```python
from build123d import *

# Parameters (mm, degrees)
SKETCH1_R                                         = 40
SKETCH1_R_2                                       = 19
BOSS_EXTRUDE1_DEPTH                               = 5
SKETCH2_R                                         = 40
SKETCH2_R_2                                       = 27
BOSS_EXTRUDE2_DEPTH                               = 4
SKETCH3_R                                         = 40
SKETCH3_R_2                                       = 32
BOSS_EXTRUDE3_DEPTH                               = 3
BOSS_EXTRUDE4_REACH                               = 92.244
BOSS_EXTRUDE4_END_RADIUS                          = 40
SKETCH6_W                                         = 12
SKETCH6_H                                         = 80
BOSS_EXTRUDE4_DIRECTION_2_DEPTH                   = 20
SKETCH9_W                                         = 60
SKETCH9_H                                         = 8
BOSS_EXTRUDE5_DEPTH                               = 82
SKETCH19_R                                        = 2.7
SKETCH19_W                                        = 18
SKETCH19_H                                        = 26
CUT_EXTRUDE8_DEPTH                                = 12
SKETCH5_R                                         = 1.4
SKETCH5_R_2                                       = 1.375
CUT_EXTRUDE1_HOLE_DEPTH                           = 149.013512897
CUT_EXTRUDE9_REALITY_DEPTH                        = 148.74302014
CUT_EXTRUDE9_REALITY_DEPTH_BACK                   = 148.74302014
CBORE_FOR_M5_HEX_HEAD_BOLT1_D                     = 5.4
CBORE_FOR_M5_HEX_HEAD_BOLT1_DEPTH                 = 17
CBORE_FOR_M5_HEX_HEAD_BOLT1_CBORE_D               = 8.4
CBORE_FOR_M5_HEX_HEAD_BOLT1_CBORE_DEPTH           = 5
CSK_FOR_M2_5_FLAT_HEAD_MACHINE_SCREW1_D           = 2.8
CSK_FOR_M2_5_FLAT_HEAD_MACHINE_SCREW1_CSINK_D     = 5.1
CSK_FOR_M2_5_FLAT_HEAD_MACHINE_SCREW1_CSINK_ANGLE = 90
FILLET1_5MM_R                                     = 5
FILLET2_2MM_R                                     = 2
FILLET3_1MM_R                                     = 1


with BuildPart() as part:
    # Sketch1 → Boss-Extrude1 (new body)
    with BuildSketch(Plane(origin=(0, 0, 0), x_dir=(1, 0, 0), z_dir=(0, 1, 0))):
        with Locations(Location((0, 0, 0), (0, 0, 270))):
            Circle(SKETCH1_R)
        with Locations(Location((0, 0, 0), (0, 0, 270))):
            Circle(SKETCH1_R_2, mode=Mode.SUBTRACT)
    extrude(amount=BOSS_EXTRUDE1_DEPTH)

    # Sketch2 → Boss-Extrude2 (add)
    with BuildSketch(Plane(origin=(0, 5, 0), x_dir=(1, 0, 0), z_dir=(0, 1, 0))):
        with Locations(Location((0, 0, 0), (0, 0, 270))):
            Circle(SKETCH2_R)
        with Locations(Location((0, 0, 0), (0, 0, 270))):
            Circle(SKETCH2_R_2, mode=Mode.SUBTRACT)
    extrude(amount=BOSS_EXTRUDE2_DEPTH)

    # Sketch3 → Boss-Extrude3 (add)
    with BuildSketch(Plane(origin=(0, 9, 0), x_dir=(1, 0, 0), z_dir=(0, 1, 0))):
        with Locations(Location((0, 0, 0), (0, 0, 270))):
            Circle(SKETCH3_R)
        with Locations(Location((0, 0, 0), (0, 0, 270))):
            Circle(SKETCH3_R_2, mode=Mode.SUBTRACT)
    extrude(amount=BOSS_EXTRUDE3_DEPTH)

    # Boss-Extrude4: up to this cylinder (the profile starts outside it)
    boss_extrude4_end = Plane(origin=(0, 6, 0), z_dir=(0, -1, 0)) * Cylinder(BOSS_EXTRUDE4_END_RADIUS, 265.488, mode=Mode.PRIVATE)
    # Sketch6 → Boss-Extrude4 (add, up to the surface)
    with BuildSketch(Plane(origin=(-40, 0, 0), x_dir=(0, -1, 0), z_dir=(-1, 0, 0)), mode=Mode.PRIVATE) as boss_extrude4_sk1:
        with Locations((-6, 0)):
            Rectangle(SKETCH6_W, SKETCH6_H)
    boss_extrude4_tool1 = extrude(boss_extrude4_sk1.sketch, amount=-BOSS_EXTRUDE4_REACH, mode=Mode.PRIVATE) - boss_extrude4_end
    add(boss_extrude4_tool1.solids().sort_by_distance((-40, 6, 0))[0])
    add(boss_extrude4_tool1.solids().sort_by_distance((-40, 6, 0))[1])

    # Sketch6 → Boss-Extrude4 direction 2 (add)
    with BuildSketch(Plane(origin=(-40, 0, 0), x_dir=(0, -1, 0), z_dir=(-1, 0, 0))):
        with Locations((-6, 0)):
            Rectangle(SKETCH6_W, SKETCH6_H)
    extrude(amount=BOSS_EXTRUDE4_DIRECTION_2_DEPTH)

    # Sketch9 → Boss-Extrude5 (add)
    with BuildSketch(Plane.ZY.offset(60)):
        with Locations((0, 4)):
            Rectangle(SKETCH9_W, SKETCH9_H)
    extrude(amount=BOSS_EXTRUDE5_DEPTH)

    # Sketch19 → Cut-Extrude8 (cut)
    with BuildSketch(Plane.XZ):
        with Locations(Location((-131.5, 15, 0), (0, 0, 270))):
            Circle(SKETCH19_R)
        with Locations(Location((-131.5, -15, 0), (0, 0, 270))):
            Circle(SKETCH19_R)
        with Locations((-44, 15)):
            Rectangle(SKETCH19_W, SKETCH19_H)
        with Locations((-44, -15)):
            Rectangle(SKETCH19_W, SKETCH19_H)
    extrude(amount=-CUT_EXTRUDE8_DEPTH, mode=Mode.SUBTRACT)

    # Sketch5 → Cut-Extrude1-Hole (cut, through all)
    with BuildSketch(Plane(origin=(0, 12, 0), x_dir=(1, 0, 0), z_dir=(0, 1, 0))):
        with Locations(Location((-0.253069529, 28.998895769, 0), (0, 0, 270))):
            Circle(SKETCH5_R)
        with Locations(Location((20.46369256, 12.05403612, 0), (0, 0, 270))):
            Circle(SKETCH5_R_2)
        with Locations(Location((20.670947779, -11.695059552, 0), (0, 0, 270))):
            Circle(SKETCH5_R_2)
        with Locations(Location((0.253069529, -28.998895769, 0), (0, 0, 270))):
            Circle(SKETCH5_R)
        with Locations(Location((-20.46369256, -12.05403612, 0), (0, 0, 270))):
            Circle(SKETCH5_R_2)
        with Locations(Location((-20.670947779, 11.695059552, 0), (0, 0, 270))):
            Circle(SKETCH5_R_2)
    extrude(amount=-CUT_EXTRUDE1_HOLE_DEPTH, mode=Mode.SUBTRACT)

    # Sketch22 → Cut-Extrude9-Reality (cut, two sides: drawn at the far end of the back side and taken through both)
    with BuildSketch(Plane(origin=(0, 8, 0), x_dir=(1, 0, 0), z_dir=(0, 1, 0)).offset(-CUT_EXTRUDE9_REALITY_DEPTH_BACK)):
        Polygon((-141.8, 29.8), (-141.8, -29.8), (-60.2, -29.8), (-60, -29.8), (-60, -30), (-142, -30), (-142, 30), (-60, 30), (-60, 29.8), (-60.2, 29.8), align=None)
    extrude(amount=CUT_EXTRUDE9_REALITY_DEPTH + CUT_EXTRUDE9_REALITY_DEPTH_BACK, mode=Mode.SUBTRACT)

    # CBORE for M5 Hex Head Bolt1
    with Locations(Plane(origin=(-131.5, 0, 15), x_dir=(0, 0, -1), z_dir=(0, -1, 0))):
        with Locations((0, 0), (30, 0)):
            CounterBoreHole(CBORE_FOR_M5_HEX_HEAD_BOLT1_D / 2, CBORE_FOR_M5_HEX_HEAD_BOLT1_CBORE_D / 2, CBORE_FOR_M5_HEX_HEAD_BOLT1_CBORE_DEPTH, depth=CBORE_FOR_M5_HEX_HEAD_BOLT1_DEPTH)

    # CSK for M2.5 Flat Head Machine Screw1 (through all)
    with Locations(Plane(origin=(-20.46369256, 0, 12.05403612), x_dir=(0, 0, -1), z_dir=(0, -1, 0))):
        with Locations((0, 0), (23.749095672, -0.207255219), (24.10807224, 40.92738512), (0.358976568, 41.134640339), (-16.944859649, 20.716762089), (41.052931889, 20.210623031)):
            CounterSinkHole(CSK_FOR_M2_5_FLAT_HEAD_MACHINE_SCREW1_D / 2, CSK_FOR_M2_5_FLAT_HEAD_MACHINE_SCREW1_CSINK_D / 2, counter_sink_angle=CSK_FOR_M2_5_FLAT_HEAD_MACHINE_SCREW1_CSINK_ANGLE)

    # Fillet1-5mm
    fillet1_5mm_edges = [part.edges().sort_by_distance(p)[0] for p in [
        (-35, 6, -2),
        (-35, 6, -28),
        (-35, 6, 28),
        (-35, 6, 2),
    ]]
    fillet(fillet1_5mm_edges, radius=FILLET1_5MM_R)

    # Fillet2-2mm
    fillet2_2mm_edges = [part.edges().sort_by_distance(p)[0] for p in [
        (40, 0, 0),
        (-30, 0, -40),
        (-30, 0, 40),
    ]]
    fillet(fillet2_2mm_edges, radius=FILLET2_2MM_R)

    # Fillet3-1mm
    fillet3_1mm_edges = [part.edges().sort_by_distance(p)[0] for p in [
        (-35, 0, -15),
        (-35, 12, -15),
        (-46.5, 0, 28),
        (-46.5, 12, 28),
        (-35, 0, 15),
        (-35, 12, 15),
        (-46.5, 0, -2),
        (-46.5, 12, -2),
        (-36.464466094, 0, -26.535533906),
        (-36.464466094, 12, -26.535533906),
        (-36.464466094, 0, 26.535533906),
        (-36.464466094, 12, 26.535533906),
        (-36.464466094, 0, 3.464466094),
        (-36.464466094, 12, 3.464466094),
        (-36.464466094, 0, -3.464466094),
        (-36.464466094, 12, -3.464466094),
        (0, 0, -19),
        (-53, 12, -15),
        (-46.5, 12, -28),
        (-53, 0, -15),
        (-46.5, 0, -28),
        (-53, 12, 15),
        (-46.5, 12, 2),
        (-53, 0, 15),
        (-46.5, 0, 2),
    ]]
    fillet(fillet3_1mm_edges, radius=FILLET3_1MM_R)


solid = part.part
```
Build history of the part. All positions in model axes, mm. A direction names the side the tool comes from. Give positions to 0.01 mm unless a question says otherwise; leave off trailing zeros. Loops run counter-clockwise (first coordinate to the right, second up) from the corner with the lowest first, then second, coordinate; pieces in that order, holes last. Notation, with made-up numbers: (-17, -13) -> (-8, -13) arc R20 cw to (-8, 8) -> close; hole circle Ø4 at (60.5, -7.75). An arc over 180 degrees is marked (long way). One line per question, with ' | ' between items.
Q1. Cut at C-C, the plane x = -103. Write the cut outline in (y, z).
Filled sheet:
outline: (0, -29.8) -> (8, -29.8) -> (8, 29.8) -> (0, 29.8) -> close
Q2. Tool access for faces 1 (the flat face through (-35, 6, -15)), 2 (the flat face through (-100, 8, 0)), 3 (the flat face through (-131, 5, -18)): list every direction of +Z, -Z, +X, -X, +Y, -Y with a clear straight run to the whole face (end or side of a thin tool).
Filled sheet:
face 1: +Y, -Y | face 2: +Z, -Z, -X, +Y | face 3: -Y
Q3. Drill centre lines: line 1 along X through (y, z) = (7.05, 0); line 2 along Z through (x, y) = (-131.5, 5.9); line 3 along Z through (x, y) = (-46.5, 9.5). Where is each one in solid material? Low to high. Write a range as [from, to].
Filled sheet:
line 1: x = [-141.8, -27], [27, 40] | line 2: z = [-29.8, -17.7], [-12.3, 12.3], [17.7, 29.8] | line 3: z = [-40, -28], [-2, 2], [28, 40]
Q4. Drop flat-ended pins along their axis: pin 1 (9 mm diameter, centred on x = -130, z = -13, fed in from -Y); pin 2 (12 mm diameter, centred on x = -42, z = -15.5, fed in from +Y); pin 3 (4.5 mm diameter, centred on x = -20.46, z = 12.05, fed in from -Y); pin 4 (6 mm diameter, centred on x = -65, y = 2, fed in from +Z). Give the stop position or say it passes through.
Filled sheet:
pin 1: stops at y = 0 | pin 2: passes through | pin 3: stops at y = 0.29 | pin 4: stops at z = 29.8
Q5. Cut at B-B, the plane x = -48. Write the cut outline in (y, z), plus the area to 3 significant figures.
Filled sheet:
outline: (0, -38) arc R2 ccw to (2, -40) -> (12, -40) -> (12, -29) arc R1 ccw to (11, -28) -> (1, -28) arc R1 ccw to (0, -29) -> close; (0, -1) arc R1 ccw to (1, -2) -> (11, -2) arc R1 ccw to (12, -1) -> (12, 1) arc R1 ccw to (11, 2) -> (1, 2) arc R1 ccw to (0, 1) -> close; (0, 29) arc R1 ccw to (1, 28) -> (11, 28) arc R1 ccw to (12, 29) -> (12, 40) -> (2, 40) arc R2 ccw to (0, 38) -> close | area: 333 mm²
Q6. Cut at A-A, the plane x = -131.5. Write the cut outline in (y, z), plus the area to 3 significant figures.
Filled sheet:
outline: (0, -29.8) -> (8, -29.8) -> (8, -17.7) -> (5, -17.7) -> (5, -19.2) -> (0, -19.2) -> close; (0, -10.8) -> (5, -10.8) -> (5, -12.3) -> (8, -12.3) -> (8, 12.3) -> (5, 12.3) -> (5, 10.8) -> (0, 10.8) -> close; (0, 19.2) -> (5, 19.2) -> (5, 17.7) -> (8, 17.7) -> (8, 29.8) -> (0, 29.8) -> close | area: 360 mm²
Q7. Pull direction X, two halves, no side cores. Call faces 4 (the flat face through (-47, 6, 28)), 5 (the cylindrical face through (39.99, 6.93, 0.88)), 6 (the flat face through (-100, 4, 29.8)): pulls with the +X half, pulls with the -X half, needs draft (parallel to the pull), parting line crosses it, or undercut.
Filled sheet:
face 4: undercut | face 5: pulls with the +X half | face 6: needs draft
